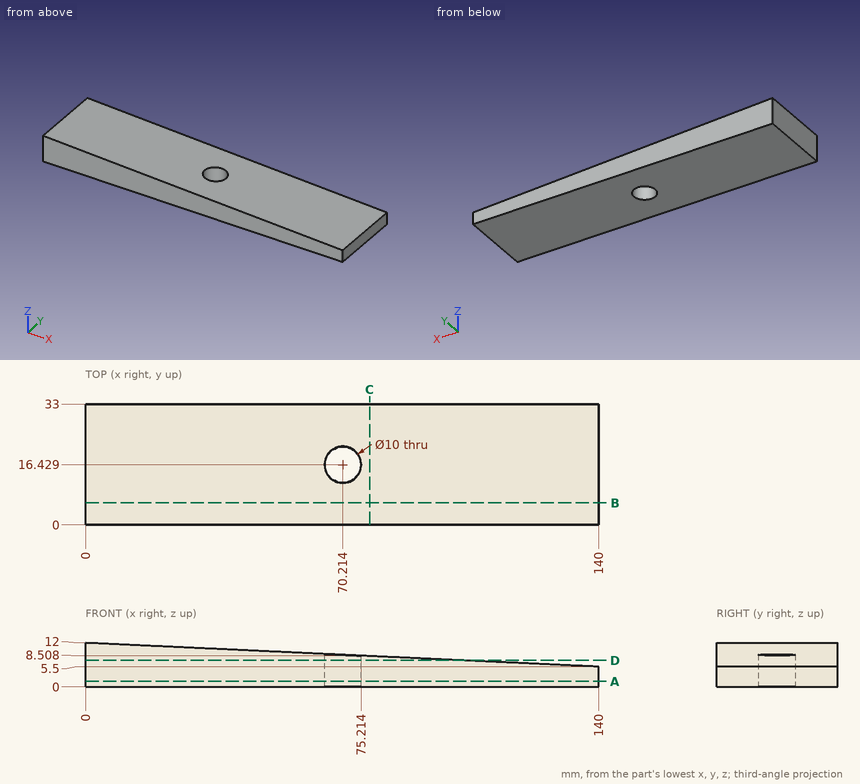
Verification items for this drawing (mm, ordinates from the low corner). Coordinates: 2 decimals unless noted, no trailing zeros. Write each loop counter-clockwise with the first axis right and the second up, starting at its lowest first coordinate (ties: lowest second). Pieces come first, ordered by that corner, then holes. Notation, with made-up numbers: (-38.5, 37.5) -> (-5.5, 37.5) arc R10 ccw to (-5.5, 43.5) -> close; hole circle Ø6 at (-11, 61.25). An arc over 180 degrees is marked (long way). Use CSV: the item, a comma, the result in double quotes. Start each with the question number.
Item 1: Cross-section at C-C, the plane x = 77.5. Record the cut outline in (y, z), plus the area to 3 significant figures.
Item 2: Thickness scan on line 1 (X direction, y = 16, z = 3.25); line 2 (Z direction, x = 65.5, y = 5); line 3 (X direction, y = 14.5, z = 3). Record the ranges inside material, lowest first.
Item 3: Cross-section at A-A, the plane z = 1.5. Record the cut outline in (x, y) (1 decimal), plus the area to 3 significant figures.
Item 4: Depth check by flat-ended pin: pin 1 Ø6 at (x, y) = (23, 11.5) entering from -Z. Enter the tip coordinate at first touch or a pass-through.
Item 5: Cross-section at B-B, the plane y = 6. Record the cut outline in (x, z), plus the area to 4 significant figures.
Item 6: Cross-section at D-D, the plane z = 7.25. Record the cut outline in (x, y) (1 decimal).
Answers:
1,outline,"(0, 0) -> (33, 0) -> (33, 8.4) -> (0, 8.4) -> close"
1,area,"277 mm^2"
2,line 1,"0 to 65.23, 75.2 to 140"
2,line 2,"0 to 8.96"
2,line 3,"0 to 65.6, 74.83 to 140"
3,outline,"(0, 0) -> (140, 0) -> (140, 33) -> (0, 33) -> close; hole circle Ø10 at (70.2, 16.4)"
3,area,"4,540 mm^2"
4,pin 1,"z = 0"
5,outline,"(0, 0) -> (140, 0) -> (140, 5.5) -> (0, 12) -> close"
5,area,"1,225 mm^2"
6,outline,"(0, 0) -> (102.3, 0) -> (102.3, 33) -> (0, 33) -> close; hole circle Ø10 at (70.2, 16.4)"
